from build123d import *

# Parameters (mm, degrees)
SKETCH1_R               = 5.35
BOSS_EXTRUDE2_DEPTH     = 7
BOSS_EXTRUDE3_START     = 8
SKETCH3_R               = 5.35
BOSS_EXTRUDE3_DEPTH     = 8
BOSS_EXTRUDE4_DEPTH     = 3
CHAMFER1_SIZE           = 10
CHAMFER2_SIZE           = 5
CUT_EXTRUDE1_DEPTH      = 67.560662475
CUT_EXTRUDE1_DEPTH_BACK = 67.560662475
SKETCH5_W               = 28.474956737
SKETCH5_H               = 3.5
SKETCH5_H_2             = 8
CHAMFER3_SIZE           = 7
SKETCH6_R               = 11
BOSS_EXTRUDE5_DEPTH     = 5
SKETCH8_W               = 3
SKETCH8_H               = 7.519820499
SKETCH8_H_2             = 11.230179501
CUT_EXTRUDE2_DEPTH      = 5
CUT_EXTRUDE3_REACH      = 91.372
SKETCH9_W               = 8
SKETCH9_H               = 4
SKETCH10_R              = 3.1
CUT_EXTRUDE4_DEPTH      = 4
SKETCH11_R              = 3.1
CUT_EXTRUDE5_DEPTH      = 1
CHAMFER4_SIZE           = 1
FILLET1_R               = 0.5


# Some blends are built 0.0001 mm under size
with BuildPart() as part:
    # Sketch1 → Boss-Extrude2 (new body)
    with BuildSketch(Plane.XY):
        Polygon((-19.503784034, -20), (19.503784034, -20), (19.503784034, -18.25), (62.978740771, -18.25), (62.978740771, 13), (19.503784034, 13), (19.503784034, 20), (-19.503784034, 20), align=None)
        Circle(SKETCH1_R, mode=Mode.SUBTRACT)
    extrude(amount=-BOSS_EXTRUDE2_DEPTH)

    # Sketch3 → Boss-Extrude3 (add)
    with BuildSketch(Plane.XY.offset(BOSS_EXTRUDE3_START)):
        with BuildLine():
            Line((7.668115805, 5.35), (62.978740771, 5.35))
            Line((62.978740771, 5.35), (62.978740771, 9.35))
            Line((62.978740771, 9.35), (0, 9.35))
            ThreePointArc((0, 9.35), (-9.35, 0), (0, -9.35))
            Line((0, -9.35), (62.978740771, -9.35))
            Line((62.978740771, -9.35), (62.978740771, -5.35))
            Line((62.978740771, -5.35), (7.668115805, -5.35))
            ThreePointArc((7.668115805, -5.35), (9.35, 0), (7.668115805, 5.35))
        make_face()
        Circle(SKETCH3_R, mode=Mode.SUBTRACT)
    extrude(amount=-BOSS_EXTRUDE3_DEPTH)

    # Sketch4 → Boss-Extrude4 (add)
    with BuildSketch(Plane.XY):
        with BuildLine():
            Line((0, -18.25), (62.978740771, -18.25))
            Line((62.978740771, -18.25), (62.978740771, -17.25))
            Line((62.978740771, -17.25), (8.306623863, -17.25))
            Line((8.306623863, -17.25), (0, -17.25))
            ThreePointArc((0, -17.25), (-17.25, 0), (0, 17.25))
            Line((0, 17.25), (0, 18.25))
            ThreePointArc((0, 18.25), (-18.25, 0), (0, -18.25))
        make_face()
    extrude(amount=BOSS_EXTRUDE4_DEPTH)

    # Chamfer1
    # the kernel refuses this chamfer: 10 mm, written as the material it takes off along each edge
    with BuildSketch(Plane(origin=(19.503784034, -20, 25.71682988), x_dir=(-0.9996219169112968, -0.027495876610586317, 0), z_dir=(0, 0, -1))) as chamfer1_piece_1_section:
        Polygon((CHAMFER1_SIZE * 0.999621916911, CHAMFER1_SIZE * 0.0274958766106), (-CHAMFER1_SIZE * 0.0274958766106, CHAMFER1_SIZE * 0.999621916911), (0, 0), align=None)
    chamfer1_piece_1 = extrude(amount=58.433659759, mode=Mode.PRIVATE)
    chamfer1_piece_1 = split(chamfer1_piece_1, bisect_by=Plane(origin=(14.814200223, -18.25, -3.5), z_dir=(0, -1, 0)), keep=Keep.TOP, mode=Mode.PRIVATE)
    add(chamfer1_piece_1, mode=Mode.SUBTRACT)

    # Chamfer2
    chamfer2_edges = [part.edges().sort_by_distance(p)[0] for p in [
        (-19.503784034, -20, -3.5),
        (-19.503784034, 20, -3.5),
    ]]
    chamfer(chamfer2_edges, length=CHAMFER2_SIZE)

    # Sketch5 → Cut-Extrude1 (cut, two sides: drawn at the far end of the back side and taken through both)
    with BuildSketch(Plane.XY.offset(-CUT_EXTRUDE1_DEPTH_BACK)):
        with Locations((38.741262403, 3.6)):
            Rectangle(SKETCH5_W, SKETCH5_H)
        with Locations((38.741262403, -7.15)):
            Rectangle(SKETCH5_W, SKETCH5_H_2)
    extrude(amount=CUT_EXTRUDE1_DEPTH + CUT_EXTRUDE1_DEPTH_BACK, mode=Mode.SUBTRACT)

    # Chamfer3
    chamfer3_edges = [part.edges().sort_by_distance(p)[0] for p in [
        (19.503784034, 20, -3.5),
    ]]
    chamfer(chamfer3_edges, length=CHAMFER3_SIZE - 0.0001)  # a hair under: the kernel refuses the full size


with BuildPart() as body_2:
    # Mirror9: mirrored copy
    add(part.part.mirror(Plane.XY.offset(-10)))

    # Sketch6 → Boss-Extrude5 (add)
    with BuildSketch(Plane.XY.offset(-13)):
        Circle(SKETCH6_R)
    extrude(amount=BOSS_EXTRUDE5_DEPTH)

    # Sketch8 → Cut-Extrude2 (cut)
    with BuildSketch(Plane(origin=(62.978740771, 0, 0), x_dir=(0, 0, -1), z_dir=(1, 0, 0))):
        with Locations((16.5, 6.240089751)):
            Rectangle(SKETCH8_W, SKETCH8_H)
        with Locations((16.5, -9.13491025)):
            Rectangle(SKETCH8_W, SKETCH8_H_2)
    extrude(amount=-CUT_EXTRUDE2_DEPTH, mode=Mode.SUBTRACT)

    # Sketch9 → Cut-Extrude3 (cut, up to next)
    with BuildSketch(Plane(origin=(62.978740771, 0, 0), x_dir=(0, 0, -1), z_dir=(1, 0, 0)), mode=Mode.PRIVATE) as cut_extrude3_sk1:
        with Locations((24, -7.35)):
            Rectangle(SKETCH9_W, SKETCH9_H)
    cut_extrude3_tool1 = extrude(cut_extrude3_sk1.sketch, amount=-CUT_EXTRUDE3_REACH, mode=Mode.PRIVATE) & body_2.part
    add(cut_extrude3_tool1.solids().sort_by_distance((62.978741, -7.35, -24))[0], mode=Mode.SUBTRACT)

    # Sketch10 → Cut-Extrude4 (cut)
    with BuildSketch(Plane(origin=(0, 0, -20), x_dir=(-1, 0, 0), z_dir=(0, 0, -1))):
        with Locations((-20.003784034, 0)):
            Circle(SKETCH10_R)
    extrude(amount=-CUT_EXTRUDE4_DEPTH, mode=Mode.SUBTRACT)

    # Sketch11 → Cut-Extrude5 (cut)
    with BuildSketch(Plane.XY.offset(-13)):
        with Locations(Location((20.003784034, 0, 0), (0, 0, 180))):
            Circle(SKETCH11_R)
    extrude(amount=-CUT_EXTRUDE5_DEPTH, mode=Mode.SUBTRACT)

    # Chamfer4
    chamfer4_edges = [body_2.edges().sort_by_distance(p)[0] for p in [
        (23.103784034, 0, -14),
    ]]
    chamfer(chamfer4_edges, length=CHAMFER4_SIZE - 0.0001)  # a hair under: the kernel refuses the full size

    # Fillet1
    fillet1_edges = [body_2.edges().sort_by_distance(p)[0] for p in [
        (0, 18.25, -21.5),
        (0, 17.25, -21.5),
    ]]
    fillet(fillet1_edges, radius=FILLET1_R - 0.0001)  # a hair under: the kernel refuses the full size


solid = body_2.part
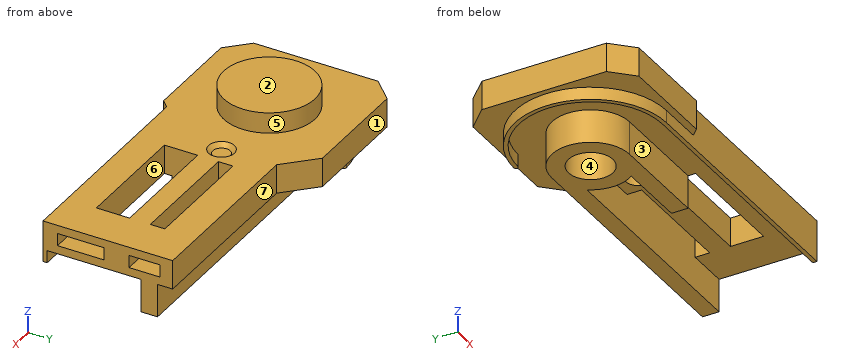
For this review, take the finished solid that the model builds, in its own axes (mm). Face numbers are marked on the shaded views. A direction names the side the tool comes from. Round coordinates to 2 decimals unless told otherwise and drop trailing zeros. Write each loop counter-clockwise with the first axis right and the second up, starting at its lowest first coordinate (ties: lowest second). Pieces come first, ordered by that corner, then holes. Notation, with made-up numbers: M 83.25,-21.75 L 113.25,-21.75 A29 cw 113.25,13.25 Z; hole C 10,15 d5. An arc over 180 degrees is marked long. Write item = value, one per line. Start each with the question number.
(1) Clearance check with flat-ended pins moving along their axes: pin 1 Ø0.9 at (x, z) = (60.5, -17) entering from +Y; pin 2 Ø10 at (x, y) = (36, 10) entering from +Z; pin 3 Ø8 at (x, z) = (15.5, -25.5) entering from -Y. State where each tip first meets the part, or that it passes through.
(2) We need section D-D (x = 3.5). Give the boundary of the cut face in (y, z).
(3) We need section C-C (y = 7.5). Give the boundary of the cut face in (x, z).
(4) For the marked faces 4, 5, 6 and 7, list the 3-axis set-ups (+Z, -Z, +X, -X, +Y, -Y) from which the entire face can be reached by the end or side of a thin tool; tool diameter is ignored.
(5) The part is to be moulded in two halves that separate along Y. For the marked faces 1, 2 and 3, say which applies: +Y half, -Y half, draft (parallel to the pull), parting line (faces both ways), or undercut.
(6) We need section B-B (x = -13.5). Give the boundary of the cut face in (y, z), then the cut area to 3 significant figures.
(7) For line 1 along Y through (x, z) = (40.5, -15.25); line 2 along Y through (x, z) = (35, -20.25); line 3 along Y through (x, z) = (20, -24), list the stretches that pass through material, from the lowest coordinate up.
Results found:
q1.pin_1 = 13
q1.pin_2 = -13
q1.pin_3 = -18.25
q2.outline = M -20,-20 L -18.25,-20 L -18.25,-23 L -17.25,-23 L -17.25,-20 L -9.35,-20 L -9.35,-28 L -4.05,-28 L -4.05,-13 L 4.05,-13 L 4.05,-28 L 9.35,-28 L 9.35,-20 L 20,-20 L 20,-13 L 10.43,-13 L 10.43,-8 L -10.43,-8 L -10.43,-13 L -20,-13 Z
q3.outline = M -19.5,-20 L -16.64,-20 L -16.64,-23 L -15.53,-23 L -15.53,-20 L -5.58,-20 L -5.58,-28 L 62.98,-28 L 62.98,-18 L 57.98,-18 L 57.98,-15 L 62.98,-15 L 62.98,-13 L 8.05,-13 L 8.05,-8 L -8.05,-8 L -8.05,-13 L -19.5,-13 Z
q4.face_4 = -Z
q4.face_5 = +Z
q4.face_6 = +Z, -Z
q4.face_7 = +Z, -Z, +X, +Y
q5.face_1 = +Y half
q5.face_2 = draft
q5.face_3 = undercut
q6.outline = M -20,-20 L -12.28,-20 L -12.28,-23 L -10.74,-23 L -10.74,-20 L 10.74,-20 L 10.74,-23 L 12.28,-23 L 12.28,-20 L 20,-20 L 20,-13 L -20,-13 Z
q6.area = 289 mm²
q7.line_1 = -18.25 to -11.15, -3.15 to 1.85, 5.35 to 13
q7.line_2 = -18.25 to -17.25, 5.35 to 9.35
q7.line_3 = -9.35 to -5.35, 5.35 to 9.35
